from build123d import *

# Parameters (mm, degrees)
SKETCH1_R           = 2
BOSS_EXTRUDE1_DEPTH = 3.5
BOSS_EXTRUDE2_START = 3.5
SKETCH1_3_R         = 2
BOSS_EXTRUDE2_DEPTH = 10
CHAMFER1_SIZE       = 0.5


with BuildPart() as part:
    # Sketch1 → Boss-Extrude1 (new body)
    with BuildSketch(Plane(origin=(0, 0, 0), x_dir=(1, 0, 0), z_dir=(0, 1, 0))):
        Polygon((-4.041451884, 0), (-2.020725942, -3.5), (2.020725942, -3.5), (4.041451884, 0), (2.020725942, 3.5), (-2.020725942, 3.5), align=None)
        Circle(SKETCH1_R, mode=Mode.SUBTRACT)
        Circle(SKETCH1_R)
    extrude(amount=BOSS_EXTRUDE1_DEPTH)

    # Sketch1<3> → Boss-Extrude2 (add)
    with BuildSketch(Plane(origin=(0, 0, 0), x_dir=(1, 0, 0), z_dir=(0, 1, 0)).offset(BOSS_EXTRUDE2_START)):
        with Locations(Location((0, 0, 0), (0, 0, 270))):
            Circle(SKETCH1_3_R)
    extrude(amount=BOSS_EXTRUDE2_DEPTH)

    # Chamfer1
    chamfer1_edges = [part.edges().sort_by_distance(p)[0] for p in [
        (0, 13.5, -2),
    ]]
    chamfer(chamfer1_edges, length=CHAMFER1_SIZE)


solid = part.part
For this review, take the finished solid that the model builds, in its own axes (mm). A direction names the side the tool comes from. Round coordinates to 2 decimals unless told otherwise and drop trailing zeros. Loops run counter-clockwise (first coordinate to the right, second up) from the corner with the lowest first, then second, coordinate; pieces in that order, holes last. Notation, with made-up numbers: (23.25, 31) - (61.25, 31) arc R15 ccw to (61.25, 42) - close; hole circle Ø6 at (-21.75, 79). An arc over 180 degrees is marked (long way). Answer as CSV lines item,"result".
(1) Tool access review of faces 1 (the face through (-2, 8, 0)), 2 (the face through (-3, 1.7, -1.8)): name each direction out of +Z, -Z, +X, -X, +Y, -Y from which nothing blocks a thin tool from reaching the whole face with its end or side.
Checked values:
face 1,"+Y"
face 2,"-Z, -X, +Y, -Y"
(2) Wall thickness on line 1 (Y direction, x = 3.5, z = 0.5); line 2 (Z direction, x = 0.75, y = 4); line 3 (Z direction, x = 1, y = 10.5): over which ranges is each line inside the solid? List them lowest first.
Checked values:
line 1,"y = 0 to 3.5"
line 2,"z = -1.85 to 1.85"
line 3,"z = -1.73 to 1.73"
(3) Insertion check: P1, Ø3, axis at x = -2.5, z = 1.5, coming from the +Y side; P2, Ø1, axis at y = 3, z = -2.5, coming from the +X side; P3, Ø4, axis at y = 7, z = 2.5, coming from the +X side. Each pin has a flat end and moves straight along its axis. Give the tip position at first contact, or say it passes through.
Checked values:
P1,"stops at y = 13.5"
P2,"stops at x = 2.89"
P3,"stops at x = 1.94"
(4) Consider section D-D on x = -3. Give the boundary of the cut face in (y, z).
Checked values:
outline,"(0, -1.8) - (3.5, -1.8) - (3.5, 1.8) - (0, 1.8) - close"
(5) Consider section A-A on x = 0. Give the boundary of the cut face in (y, z), then the cut area to 4 significant figures.
Checked values:
outline,"(0, -3.5) - (3.5, -3.5) - (3.5, -2) - (13, -2) - (13.5, -1.5) - (13.5, 1.5) - (13, 2) - (3.5, 2) - (3.5, 3.5) - (0, 3.5) - close"
area,"64.25 mm2"
(6) Consider section B-B on y = 7.5. Give the boundary of the cut face in (x, z).
Checked values:
outline,"circle Ø4 at (0, 0)"
(7) Consider section C-C on z = -2.5. Give the boundary of the cut face in (x, y).
Checked values:
outline,"(-2.6, 0) - (2.6, 0) - (2.6, 3.5) - (-2.6, 3.5) - close"
